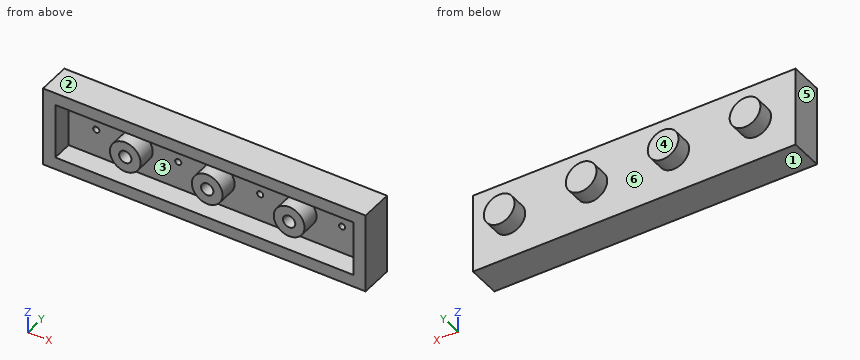
from build123d import *

# Parameters (mm, degrees)
SKETCH1_W            = 31.5
SKETCH1_H            = 3.2
BOSS_EXTRUDE1_DEPTH  = 7.8
SKETCH2_R            = 1.5
BOSS_EXTRUDE2_DEPTH  = 1.6
LPATTERN1_COUNT      = 2
LPATTERN1_PITCH      = 8
LPATTERN1_COUNT_DIR2 = 4
LPATTERN1_PITCH_DIR2 = 8
SHELL1_T             = -1.2
SKETCH3_R            = 1.5
SKETCH3_R_2          = 0.6
BOSS_EXTRUDE3_DEPTH  = 1.8
LPATTERN2_COUNT      = 3
LPATTERN2_PITCH      = 8


with BuildPart() as part:
    # Sketch1 → Boss-Extrude1 (new body)
    with BuildSketch(Plane.XY):
        with Locations((15.75, 1.6)):
            Rectangle(SKETCH1_W, SKETCH1_H)
    extrude(amount=-BOSS_EXTRUDE1_DEPTH)

    # Sketch2 → Boss-Extrude2 (add)
    with BuildSketch(Plane(origin=(0, 3.2, 0), x_dir=(1, 0, 0), z_dir=(0, 1, 0))):
        with Locations(Location((3.9, 3.9, 0), (0, 0, 270))):
            Circle(SKETCH2_R)
    boss_extrude2 = extrude(amount=BOSS_EXTRUDE2_DEPTH)

    # LPattern1: Boss-Extrude2 2 × 4, 4 skipped
    with Locations(*[(j * LPATTERN1_PITCH_DIR2, 0, i * LPATTERN1_PITCH) for i in range(LPATTERN1_COUNT) for j in range(LPATTERN1_COUNT_DIR2) if (i, j) not in ((0, 0), (1, 0), (1, 1), (1, 2), (1, 3))]):
        add(boss_extrude2)

    # Shell1
    shell1_openings = [part.faces().sort_by_distance(p)[0] for p in [
        (15.75, 0, -3.9),
    ]]
    offset(amount=SHELL1_T, openings=shell1_openings, kind=Kind.INTERSECTION)

    # Sketch3 → Boss-Extrude3 (add)
    with BuildSketch(Plane.XZ.offset(-2)):
        with Locations(Location((7.9, -3.9, 0), (0, 0, 90))):
            Circle(SKETCH3_R)
        with Locations(Location((7.9, -3.9, 0), (0, 0, 270))):
            Circle(SKETCH3_R_2, mode=Mode.SUBTRACT)
    boss_extrude3 = extrude(amount=BOSS_EXTRUDE3_DEPTH)

    # LPattern2: Boss-Extrude3 ×3
    with Locations(*[(i * LPATTERN2_PITCH, 0, 0) for i in range(1, LPATTERN2_COUNT)]):
        add(boss_extrude3)


solid = part.part
Work out the finished part from the listing and answer in its coordinate system (mm). Face numbers are marked on the shaded views. A direction names the side the tool comes from. Coordinates: 2 decimals unless noted, no trailing zeros. Write each loop counter-clockwise with the first axis right and the second up, starting at its lowest first coordinate (ties: lowest second). Pieces come first, ordered by that corner, then holes. Notation, with made-up numbers: M 89.5,34 L 110.5,34 A26 cw 110.5,59 Z; hole C 86,-4.5 d8. An arc over 180 degrees is marked long. Use one line per item in the form item = value. Start each with the question number.
1. Straight lines are drawn through the part: probe 1 along X at (y, z) = (2.6, -3.9); probe 2 along X at (y, z) = (1, -5.75); probe 3 along Z at (x, y) = (8, 0.9). For each, find the intervals that lie inside material, in ascending order. Write a range as from..to.
2. The mould has two halves that part along Z. Classify the marked faces 1, 2, 3 and 4: released by +Z, released by -Z, zero draft, split by the parting line, or undercut.
3. Each of these flat-tipped pins is pushed along its axis until it touches: P1, Ø2.5, axis at x = 8.5, z = -4.5, coming from the -Y side; P2, Ø0.7, axis at x = 4, z = -4, coming from the -Y side; P3, Ø1, axis at x = 14.5, z = -4, coming from the +Y side. Where does it stop, or does it pass through?
4. The part is cut by section A-A (x = 27.9). Give the vertices of the cut face in (y, z), plus the area to 3 significant figures.
5. The part is cut by section B-B (x = 23.9). Give the vertices of the cut face in (y, z).
6. A tool of negligible diameter and unlimited length cuts with its end or side. For the marked faces 5 and 6, from which of +Z, -Z, +X, -X, +Y, -Y can it reach the whole face along a straight path? Write none if from no direction.
Evaluation:
q1.probe_1 = 0..3.6, 4.2..11.6, 12.2..19.6, 20.2..27.6, 28.2..31.5
q1.probe_2 = 0..1.2, 30.3..31.5
q1.probe_3 = -7.8..-6.6, -5.4..-4.49, -3.31..-2.4, -1.2..0
q2.face_1 = released by -Z
q2.face_2 = released by +Z
q2.face_3 = undercut
q2.face_4 = zero draft
q3.P1 = 0.2
q3.P2 = 2
q3.P3 = 3.2
q4.outline = M 0,-7.8 L 3.2,-7.8 L 3.2,-5.4 L 4.8,-5.4 L 4.8,-2.4 L 3.2,-2.4 L 3.2,0 L 0,0 L 0,-1.2 L 2,-1.2 L 2,-3.6 L 3.6,-3.6 L 3.6,-4.2 L 2,-4.2 L 2,-6.6 L 0,-6.6 Z
q4.area = 18.0 mm^2
q5.outline = M 0,-7.8 L 3.2,-7.8 L 3.2,0 L 0,0 L 0,-1.2 L 2,-1.2 L 2,-2.4 L 0.2,-2.4 L 0.2,-3.3 L 2,-3.3 L 2,-4.5 L 0.2,-4.5 L 0.2,-5.4 L 2,-5.4 L 2,-6.6 L 0,-6.6 Z
q6.face_5 = +Z, -Z, -X, +Y, -Y
q6.face_6 = +Y
